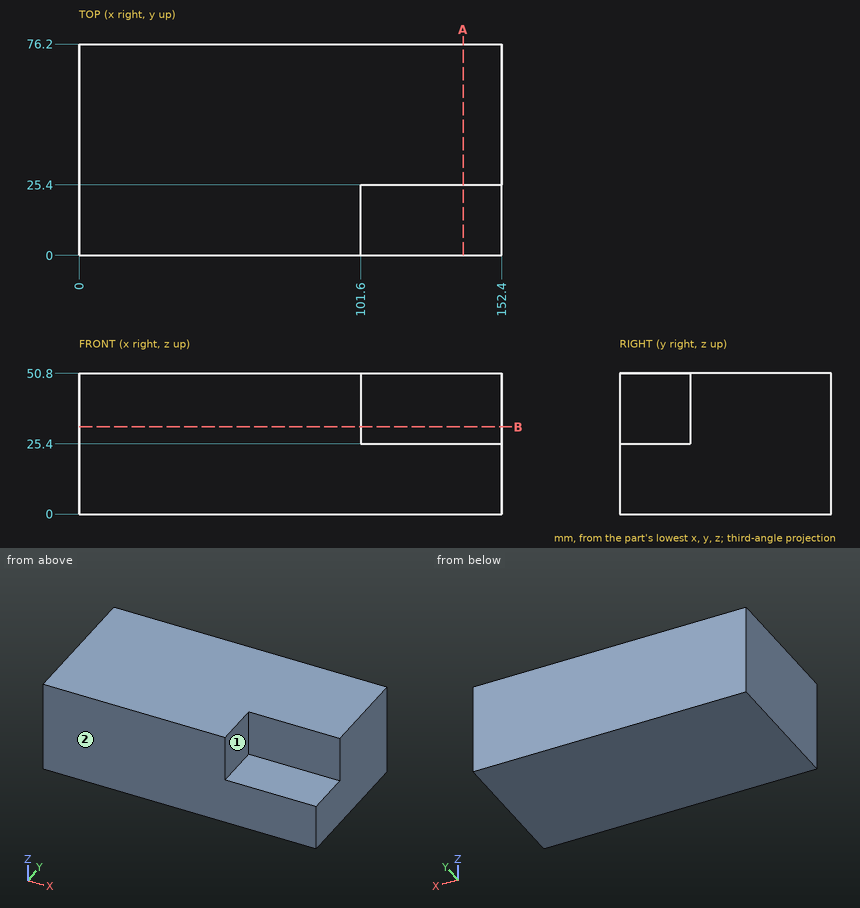
Drawing for the job (mm, zero at the part's lowest x, y, z). A direction names the side the tool comes from. Give positions to 0.01 mm unless a question says otherwise; leave off trailing zeros. Order: outer loops, then holes, each group sorted by start corner. A loop starts at its lowest first (then second) coordinate and runs counter-clockwise, first axis right, second up. Notation, with made-up numbers: M 4.5,-39 L 62.5,-39 A14 ccw 62.5,-22 Z; hole C 1.5,-27.75 d8. An arc over 180 degrees is marked long. Use a Markdown table: item, result. Add a question column.
(1) Drop flat-ended pins along their axis: P1, Ø1, axis at x = 102.5, y = 15.5, coming from the -Z side; P2, Ø12.5, axis at x = 138.5, y = 9.5, coming from the +Z side; P3, Ø12.5, axis at x = 128, z = 35, coming from the -Y side. Give the stop position or say it passes through.
(2) Saw through at A-A, the plane x = 138.5. Give the cut face in (y, z).
(3) 3-axis set-ups, long thin cutter, end or side, ignore diameter. For the marked faces 1 and 2: which of +Z, -Z, +X, -X, +Y, -Y reach the whole face in a straight line?
(4) Saw through at B-B, the plane z = 31.5. Give the cut face in (x, y), and give its area (3 significant figures).
(5) Probe line 1 along X through (y, z) = (17, 35); line 2 along Y through (x, z) = (143, 46.5). List the from-to ranges inside material, lowest first. Write a range as [from, to].
Answer key:
| question | item | result |
|---|---|---|
| 1 | P1 | z = 0 |
| 1 | P2 | z = 25.4 |
| 1 | P3 | y = 25.4 |
| 2 | outline | M 0,0 L 76.2,0 L 76.2,50.8 L 25.4,50.8 L 25.4,25.4 L 0,25.4 Z |
| 3 | face 1 | +Z, +X, -Y |
| 3 | face 2 | +Z, -Z, +X, -X, -Y |
| 4 | outline | M 0,0 L 101.6,0 L 101.6,25.4 L 152.4,25.4 L 152.4,76.2 L 0,76.2 Z |
| 4 | area | 10,300 mm^2 |
| 5 | line 1 | [0, 101.6] |
| 5 | line 2 | [25.4, 76.2] |
